CAD build for the part. Positions are in the model's coordinates, mm. A direction names the side the tool comes from. Round coordinates to 2 decimals unless told otherwise and drop trailing zeros. Loops run counter-clockwise (first coordinate to the right, second up) from the corner with the lowest first, then second, coordinate; pieces in that order, holes last.
from build123d import *

# Parameters (mm, degrees)
SKETCH1_W           = 135
SKETCH1_H           = 80
BOSS_EXTRUDE1_DEPTH = 3.5
SKETCH2_R           = 21
BOSS_EXTRUDE2_DEPTH = 13
CUT_EXTRUDE1_DEPTH  = 80.531440324
FILLET1_R           = 6
FILLET2_R           = 4.5


with BuildPart() as part:
    # Sketch1 → Boss-Extrude1 (new body)
    with BuildSketch(Plane(origin=(0, 0, 0), x_dir=(1, 0, 0), z_dir=(0, 1, 0))):
        Rectangle(SKETCH1_W, SKETCH1_H)
    extrude(amount=BOSS_EXTRUDE1_DEPTH)

    # Sketch2 → Boss-Extrude2 (add)
    with BuildSketch(Plane(origin=(0, 3.5, 0), x_dir=(1, 0, 0), z_dir=(0, 1, 0))):
        with Locations(Location((0, 0, 0), (0, 0, 90))):
            Circle(SKETCH2_R)
    extrude(amount=BOSS_EXTRUDE2_DEPTH)

    # Sketch4 → Cut-Extrude1 (cut, through all)
    with BuildSketch(Plane(origin=(0, 3.5, 0), x_dir=(1, 0, 0), z_dir=(0, 1, 0))):
        Polygon((46.191495321, -26.055456352), (56.444543648, -36.308504679), (62.808504679, -29.944543648), (52.555456352, -19.691495321), align=None)
        Polygon((-56.444543648, 36.308504679), (-46.191495321, 26.055456352), (-52.555456352, 19.691495321), (-62.808504679, 29.944543648), align=None)
        Polygon((62.808504679, 29.944543648), (56.444543648, 36.308504679), (46.191495321, 26.055456352), (52.555456352, 19.691495321), align=None)
        Polygon((-62.808504679, -29.944543648), (-52.555456352, -19.691495321), (-46.191495321, -26.055456352), (-56.444543648, -36.308504679), align=None)
    extrude(amount=-CUT_EXTRUDE1_DEPTH, mode=Mode.SUBTRACT)

    # Fillet1
    fillet1_edges = [part.edges().sort_by_distance(p)[0] for p in [
        (67.5, 1.75, 40),
        (-67.5, 1.75, 40),
        (-67.5, 1.75, -40),
        (67.5, 1.75, -40),
    ]]
    fillet(fillet1_edges, radius=FILLET1_R)

    # Fillet2
    fillet2_edges = [part.edges().sort_by_distance(p)[0] for p in [
        (56.444543648, 1.75, -36.308504679),
        (52.555456352, 1.75, 19.691495321),
        (46.191495321, 1.75, -26.055456352),
        (46.191495321, 1.75, 26.055456352),
        (52.555456352, 1.75, -19.691495321),
        (56.444543648, 1.75, 36.308504679),
        (62.808504679, 1.75, -29.944543648),
        (62.808504679, 1.75, 29.944543648),
        (-52.555456352, 1.75, 19.691495321),
        (-46.191495321, 1.75, 26.055456352),
        (-46.191495321, 1.75, -26.055456352),
        (-52.555456352, 1.75, -19.691495321),
        (-56.444543648, 1.75, 36.308504679),
        (-62.808504679, 1.75, 29.944543648),
        (-62.808504679, 1.75, -29.944543648),
        (-56.444543648, 1.75, -36.308504679),
    ]]
    fillet(fillet2_edges, radius=FILLET2_R - 0.0001)  # a hair under: the kernel refuses the full size


solid = part.part
Item 1: Cut at D-D (y = 9). List the corners of the cut face in (x, z), plus the area to 3 significant figures.
Verdict:
outline: circle Ø42 at (0, 0)
area: 1,390 mm2
Item 2: Mould opens along Z. For faces 1 (the cylindrical face through (52.605, 1.726, 21.556)), 2 (the flat face through (0, 16.5, 0)), 3 (the cylindrical face through (-52.506, 1.726, 21.556)), 4 (the cylindrical face through (65.696, 1.774, 38.289)) say: released by +Z, released by -Z, zero draft, split by the parting line, or undercut.
Verdict:
face 1: undercut
face 2: zero draft
face 3: undercut
face 4: released by +Z
Item 3: Wall check: L1, parallel to Y at x = -44, z = -32.5; L2, parallel to Z at x = 1, y = 13; L3, parallel to Z at x = -11.5, y = 5.5. Give the ranges that are in metal, low to high.
Verdict:
L1: y = 0 to 3.5
L2: z = -20.98 to 20.98
L3: z = -17.57 to 17.57
Item 4: 3-axis set-ups, long thin cutter, end or side, ignore diameter. For faces 5 (the cylindrical face through (-65.789, 1.774, 38.196)), 6 (the cylindrical face through (60.944, 1.726, -29.994)): which of +Z, -Z, +X, -X, +Y, -Y reach the whole face in a straight line?
Verdict:
face 5: +Z, -X, +Y, -Y
face 6: +Y, -Y
Item 5: Cut at B-B (y = 2). State how many separate pieces and enclosed holes the cut face has, plus the area to 3 significant figures.
Verdict:
separate pieces: 1
enclosed holes: 4
area: 10,300 mm2
Item 6: Cut at C-C (x = -15). List the corners of the cut face in (y, z).
Verdict:
outline: (0, -40) - (3.5, -40) - (3.5, -14.7) - (16.5, -14.7) - (16.5, 14.7) - (3.5, 14.7) - (3.5, 40) - (0, 40) - close
Item 7: Cut at A-A (z = 0). List the corners of the cut face in (x, y), plus the area to 3 significant figures.
Verdict:
outline: (-67.5, 0) - (67.5, 0) - (67.5, 3.5) - (21, 3.5) - (21, 16.5) - (-21, 16.5) - (-21, 3.5) - (-67.5, 3.5) - close
area: 1,020 mm2
Item 8: Flat gauge pins, fed straight in: P1, Ø4, axis at x = 20.5, y = 8.5, coming from the -Z side; P2, Ø1.5, axis at y = 14.5, z = 23, coming from the +X side; P3, Ø6, axis at x = -6, y = 14, coming from the +Z side; P4, Ø3, axis at x = -16.5, y = 6, coming from the -Z side. Where does each tip first touch, or does it go through?
Verdict:
P1: stops at z = -9.94
P2: passes through
P3: stops at z = 20.78
P4: stops at z = -14.7
